Can you work these out from the model? Positions are in its coordinate system, mm. Face numbers are marked on the shaded views. A direction names the side the tool comes from. Give positions to 0.01 mm unless a question says otherwise; leave off trailing zeros. Order: outer loops, then holes, each group sorted by start corner. A loop starts at its lowest first (then second) coordinate and runs counter-clockwise, first axis right, second up. Notation, with made-up numbers: (40, 42) -> (50, 42) arc R17 cw to (50, 59) -> close; hole circle Ø11 at (6.25, 33). An arc over 180 degrees is marked (long way). Answer as a JSON object with one key per item and string values.
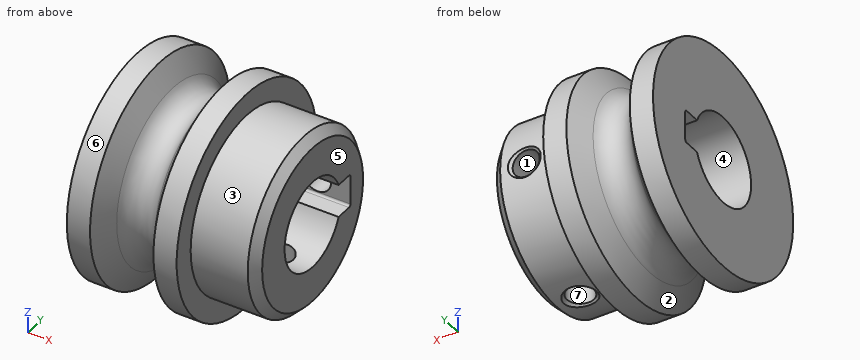
Autodesk Inventor part; units mm, degrees
ref_plane "YZ Plane" through (0, 0, 0) normal (1, 0, 0) x (0, 1, 0)
ref_plane "XZ Plane" through (0, 0, 0) normal (0, 1, 0) x (-1, 0, 0)
ref_plane "XY Plane" through (0, 0, 0) normal (0, 0, 1) x (1, 0, 0)
sketch "Sketch_2" plane through (0, 0, 0) normal (0, 0, 1) x (1, 0, 0)
  line L0 (11, 0) -> (-5, 0)
  line L1 (-5, 10) -> (-5, 4)
  line L2 (-5, 4) -> (11, 4)
  line L3 (11, 4) -> (11, 7.2)
  line L4 (11, 7.2) -> (10.2, 8)
  line L5 (10.2, 8) -> (5, 8)
  line L6 (5, 8) -> (5, 10)
  line L7 (5, 10) -> (2.8868, 10)
  line L8 (2.8868, 10) -> (1.7321, 8)
  arc A0 (-1.7321, 8) -> (1.7321, 8) centre (0, 9) ccw
  line L9 (-1.7321, 8) -> (-2.8868, 10)
  line L10 (-2.8868, 10) -> (-5, 10)
revolve "Revolution1" add sketch "Sketch_2" angle 360 about axis through (11, 0, 0) along (1, 0, 0)
sketch "Sketch_4" plane through (-5, 0, 0) normal (1, 0, 0) x (0, 0, -1)
  line L0 (-1.5, 2.6) -> (1.5, 2.6)
  line L1 (1.5, 2.6) -> (1.5, 5.2)
  arc A0 (1.5, 5.2) -> (1.3, 5.4) centre (1.3, 5.2) ccw
  line L2 (1.3, 5.4) -> (-1.3, 5.4)
  arc A1 (-1.3, 5.4) -> (-1.5, 5.2) centre (-1.3, 5.2) ccw
  line L3 (-1.5, 5.2) -> (-1.5, 2.6)
extrude "Extrusion1" cut sketch "Sketch_4" along normal blind 30
sketch "Sketch_5" plane through (0, 0, 0) normal (0, 0, 1) x (1, 0, 0)
  line L0 (8, 5.4) -> (8, 8)
  line L1 (8, 8) -> (9.5, 8)
  line L2 (9.5, 8) -> (9.2295, 7.7295)
  line L3 (9.2295, 7.7295) -> (9.2295, 5.4)
  line L4 (9.2295, 5.4) -> (8, 5.4)
  line L5 (8, 5.4) -> (8, 8)
revolve "Revolution2" cut sketch "Sketch_5" angle 360 about axis through (8, 5.4, 0) along (0, -1, 0)
thread "Thread1"
sketch "Sketch_8" plane through (0, 0, 0) normal (0, 1, 0) x (-1, 0, 0)
  line L0 (-8, -3) -> (-8, -8)
  line L1 (-8, -8) -> (-9.5, -8)
  line L2 (-9.5, -8) -> (-9.2295, -7.7295)
  line L3 (-9.2295, -7.7295) -> (-9.2295, -3)
  line L4 (-9.2295, -3) -> (-8, -3)
  line L5 (-8, -3) -> (-8, -8)
revolve "Revolution3" cut sketch "Sketch_8" angle 360 about axis through (8, 0, -3) along (0, 0, 1)
thread "Thread2"
properties part number "MBR18-2-N8"
1. If we section it at A-A on y = 0: Please give me the cut outline in (x, z).
Worked answers:
{"outline": "(-5, -10) -> (-2.89, -10) -> (-1.73, -8) arc R2 cw to (1.73, -8) -> (2.89, -10) -> (5, -10) -> (5, -8) -> (6.5, -8) -> (6.77, -7.73) -> (6.77, -4) -> (-5, -4) -> close; (-5, 4) -> (11, 4) -> (11, 7.2) -> (10.2, 8) -> (5, 8) -> (5, 10) -> (2.89, 10) -> (1.73, 8) arc R2 cw to (-1.73, 8) -> (-2.89, 10) -> (-5, 10) -> close; (9.23, -7.73) -> (9.5, -8) -> (10.2, -8) -> (11, -7.2) -> (11, -4) -> (9.23, -4) -> close"}
2. Will these pins go through, and if not, where does the flat tip stop? pin 1 Ø6 at (y, z) = (3.5, 0.5) entering from +X; pin 2 Ø4 at (x, y) = (8, -1.5) entering from +Z; pin 3 Ø1.6 at (x, y) = (5.5, 4.5) entering from +Z; pin 4 Ø6 at (x, z) = (-2, 3) entering from -Y.
Worked answers:
{"pin 1": "x = 11", "pin 2": "z = 8", "pin 3": "z = 9.22", "pin 4": "y = -10"}
3. If we section it at D-D on x = -2.25: Please give me the cut outline in (y, z).
Worked answers:
{"outline": "circle Ø17.79 at (0, 0); hole (3.71, -1.5) -> (5.2, -1.5) arc R0.2 ccw to (5.4, -1.3) -> (5.4, 1.3) arc R0.2 ccw to (5.2, 1.5) -> (3.71, 1.5) arc R4 ccw (long way) to start"}
4. If we mould it in two halves opening along Y, with no side actions, what happens to the marked faces 4, 5, 6 and 7? For each: +Y half, -Y half, draft (parallel to the pull), parting line (faces both ways), or undercut.
Worked answers:
{"face 4": "undercut", "face 5": "draft", "face 6": "parting line", "face 7": "undercut"}
5. If we section it at C-C on x = 8: Please give me the cut outline in (y, z), then the cut area to 3 significant figures.
Worked answers:
{"outline": "(-1.38, -7.88) -> (-1.23, -7.73) -> (-1.23, -3.81) arc R4 cw (long way) to (3.71, 1.5) -> (5.2, 1.5) arc R0.2 cw to (5.4, 1.3) -> (5.4, 1.23) -> (7.73, 1.23) -> (7.88, 1.38) arc R8 ccw (long way) to start; (1.23, -7.73) -> (1.38, -7.88) arc R8 ccw to (7.88, -1.38) -> (7.73, -1.23) -> (5.4, -1.23) -> (5.4, -1.3) arc R0.2 cw to (5.2, -1.5) -> (3.71, -1.5) arc R4 cw to (1.23, -3.81) -> close", "area": "130 mm²"}
6. If we section it at B-B on z = 0: Please give me the cut outline in (x, y).
Worked answers:
{"outline": "(-5, -10) -> (-2.89, -10) -> (-1.73, -8) arc R2 cw to (1.73, -8) -> (2.89, -10) -> (5, -10) -> (5, -8) -> (10.2, -8) -> (11, -7.2) -> (11, -4) -> (-5, -4) -> close; (-5, 5.4) -> (6.77, 5.4) -> (6.77, 7.73) -> (6.5, 8) -> (5, 8) -> (5, 10) -> (2.89, 10) -> (1.73, 8) arc R2 cw to (-1.73, 8) -> (-2.89, 10) -> (-5, 10) -> close; (9.23, 5.4) -> (11, 5.4) -> (11, 7.2) -> (10.2, 8) -> (9.5, 8) -> (9.23, 7.73) -> close"}
7. Please list where these lines run through material, in increasing order: L1, parallel to X at y = 0, z = -5.8; L2, parallel to Y at x = 8.75, z = -3; L3, parallel to Y at x = 6.5, z = 0.5.
Worked answers:
{"L1": "-5 to 6.77, 9.23 to 11", "L2": "-7.42 to -2.65, 2.65 to 7.42", "L3": "-7.98 to -3.97, 5.4 to 7.98"}
8. For the marked faces 1, 2 and 3, which set-ups out of +Z, -Z, +X, -X, +Y, -Y let a thin tool reach every point of the face, with its end or its side?
Worked answers:
{"face 1": "+Y", "face 2": "none", "face 3": "+X"}
